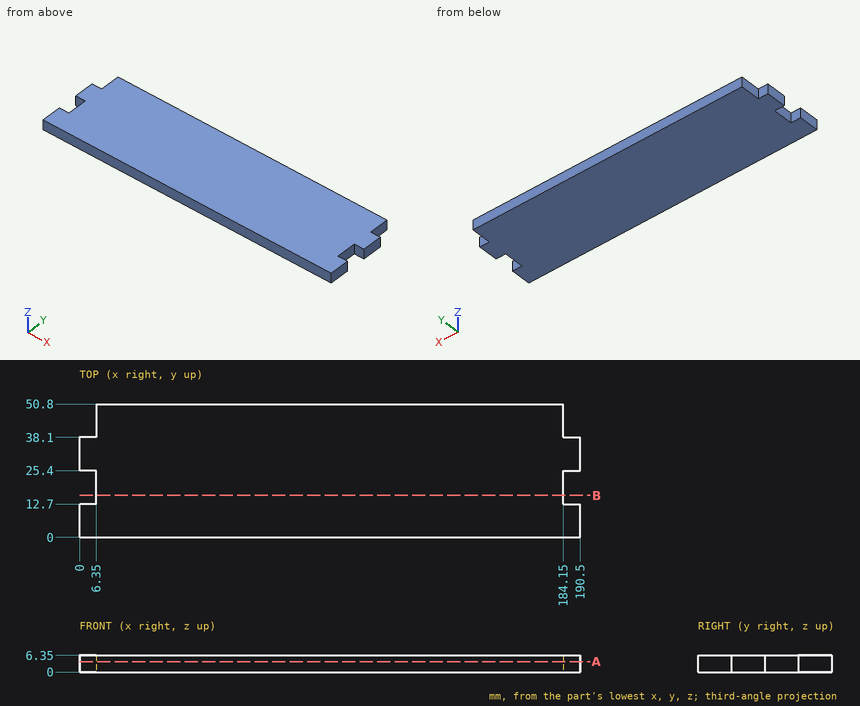
Can you work these out from the drawing? Everything is in mm from the part's minimum corner. Coordinates: 2 decimals unless noted, no trailing zeros. Loops run counter-clockwise (first coordinate to the right, second up) from the corner with the lowest first, then second, coordinate; pieces in that order, holes last. Notation, with made-up numbers: (60, -31.75) - (67, -31.75) arc R6 ccw to (67, -26.75) - close; hole circle Ø3 at (79, 29). An arc over 180 degrees is marked (long way). Use a Markdown table: item, result.
Item 1: I want a section at A-A on z = 4. Please give me the cut outline in (x, y), and give its area (3 significant figures).
Numbers:
| item | result |
|---|---|
| outline | (0, 0) - (190.5, 0) - (190.5, 12.7) - (184.15, 12.7) - (184.15, 25.4) - (190.5, 25.4) - (190.5, 38.1) - (184.15, 38.1) - (184.15, 50.8) - (6.35, 50.8) - (6.35, 38.1) - (0, 38.1) - (0, 25.4) - (6.35, 25.4) - (6.35, 12.7) - (0, 12.7) - close |
| area | 9,350 mm2 |
Item 2: Will these pins go through, and if not, where does the flat tip stop? pin 1 (3 mm diameter, centred on y = 45, z = 4.5, fed in from -X); pin 2 (3 mm diameter, centred on x = 2, z = 3, fed in from +Y).
Numbers:
| item | result |
|---|---|
| pin 1 | stops at x = 6.35 |
| pin 2 | stops at y = 38.1 |
Item 3: If I drill on probe 1 along X at (y, z) = (25, 4), over which ranges is the centre line in solid material (lowest first)? Write a range as from..to.
Numbers:
| item | result |
|---|---|
| probe 1 | x = 6.35..184.15 |
Item 4: I want a section at B-B on y = 16. Please give me the cut outline in (x, z), and give its area (3 significant figures).
Numbers:
| item | result |
|---|---|
| outline | (6.35, 0) - (184.15, 0) - (184.15, 6.35) - (6.35, 6.35) - close |
| area | 1,130 mm2 |
